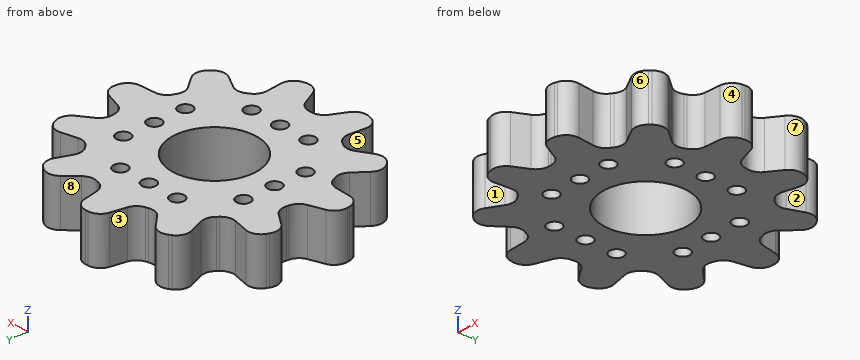
from build123d import *

# Parameters (mm, degrees)
ESBO_O1_R                = 4.5
ESBO_O1_R_2              = 0.75
RESSALTO_EXTRUS_O1_DEPTH = 5


with BuildPart() as part:
    # Esboço1 → Ressalto-extrusão1 (new body)
    with BuildSketch(Plane.XY):
        with BuildLine():
            Line((4.514334386, 10.407189323), (5.686971288, 11.63699072))
            ThreePointArc((5.686971288, 11.63699072), (6.526679908, 12.060076339), (7.444654683, 11.856522115))
            ThreePointArc((7.444654683, 11.856522115), (7.568971444, 11.77754946), (7.692450547, 11.697273382))
            ThreePointArc((7.692450547, 11.697273382), (8.258950485, 10.946813637), (8.222925837, 10.007231691))
            Line((8.222925837, 10.007231691), (7.591390112, 8.429685683))
            ThreePointArc((7.591390112, 8.429685683), (7.512037525, 7.668211946), (7.845097462, 6.978857056))
            ThreePointArc((7.845097462, 6.978857056), (7.935370531, 6.876037706), (8.024296131, 6.772050768))
            ThreePointArc((8.024296131, 6.772050768), (8.65923501, 6.344275472), (9.424251093, 6.314451352))
            Line((9.424251093, 6.314451352), (11.075616863, 6.715050749))
            ThreePointArc((11.075616863, 6.715050749), (12.010762061, 6.616992265), (12.672961861, 5.949456923))
            ThreePointArc((12.672961861, 5.949456923), (12.734847935, 5.815810182), (12.795324642, 5.681519805))
            ThreePointArc((12.795324642, 5.681519805), (12.866165546, 4.743919904), (12.327883333, 3.972969668))
            Line((12.327883333, 3.972969668), (10.94371591, 2.987287505))
            ThreePointArc((10.94371591, 2.987287505), (10.465276482, 2.389596282), (10.372770939, 1.629608249))
            ThreePointArc((10.372770939, 1.629608249), (10.39312514, 1.494305802), (10.411714532, 1.358749614))
            ThreePointArc((10.411714532, 1.358749614), (10.714586321, 0.655608259), (11.342034667, 0.216919693))
            Line((11.342034667, 0.216919693), (12.94783234, -0.338870389))
            ThreePointArc((12.94783234, -0.338870389), (13.681512123, -0.926940099), (13.877693191, -1.846518805))
            ThreePointArc((13.877693191, -1.846518805), (13.857500186, -1.992407736), (13.835773571, -2.138076166))
            ThreePointArc((13.835773571, -2.138076166), (13.388463955, -2.96513488), (12.518824975, -3.322682154))
            Line((12.518824975, -3.322682154), (10.82148923, -3.403553348))
            ThreePointArc((10.82148923, -3.403553348), (10.095864099, -3.647699318), (9.607162934, -4.237029663))
            ThreePointArc((9.607162934, -4.237029663), (9.551135951, -4.361857637), (9.493487134, -4.485944943))
            ThreePointArc((9.493487134, -4.485944943), (9.368132181, -5.241209943), (9.658802374, -5.949482436))
            Line((9.658802374, -5.949482436), (10.709202535, -7.285202572))
            ThreePointArc((10.709202535, -7.285202572), (11.008478755, -8.176575531), (10.676354988, -9.05623786))
            ThreePointArc((10.676354988, -9.05623786), (10.580494041, -9.168050275), (10.48346215, -9.278848062))
            ThreePointArc((10.48346215, -9.278848062), (9.660019656, -9.73278029), (8.735128141, -9.563405868))
            Line((8.735128141, -9.563405868), (7.263516181, -8.713790062))
            ThreePointArc((7.263516181, -8.713790062), (6.521086199, -8.526876158), (5.791348577, -8.758440595))
            ThreePointArc((5.791348577, -8.758440595), (5.676728583, -8.833162095), (5.56114465, -8.906383676))
            ThreePointArc((5.56114465, -8.906383676), (5.047362265, -9.473981021), (4.908968572, -10.226965929))
            Line((4.908968572, -10.226965929), (5.070476592, -11.918534414))
            ThreePointArc((5.070476592, -11.918534414), (4.840331165, -12.830206005), (4.085349512, -13.390665382))
            ThreePointArc((4.085349512, -13.390665382), (3.944255796, -13.432901631), (3.802725568, -13.473651259))
            ThreePointArc((3.802725568, -13.473651259), (2.864587371, -13.410336727), (2.178089842, -12.767815792))
            Line((2.178089842, -12.767815792), (1.399428066, -11.257459999))
            ThreePointArc((1.399428066, -11.257459999), (0.875909507, -10.698830065), (0.136821968, -10.499108522))
            ThreePointArc((0.136821968, -10.499108522), (0, -10.5), (-0.136821968, -10.499108522))
            ThreePointArc((-0.136821968, -10.499108522), (-0.875909507, -10.698830065), (-1.399428066, -11.257459999))
            Line((-1.399428066, -11.257459999), (-2.178089842, -12.767815792))
            ThreePointArc((-2.178089842, -12.767815792), (-2.864587371, -13.410336727), (-3.802725568, -13.473651259))
            ThreePointArc((-3.802725568, -13.473651259), (-3.944255796, -13.432901631), (-4.085349512, -13.390665382))
            ThreePointArc((-4.085349512, -13.390665382), (-4.840331165, -12.830206005), (-5.070476592, -11.918534414))
            Line((-5.070476592, -11.918534414), (-4.908968572, -10.226965929))
            ThreePointArc((-4.908968572, -10.226965929), (-5.047362265, -9.473981021), (-5.56114465, -8.906383676))
            ThreePointArc((-5.56114465, -8.906383676), (-5.676728583, -8.833162095), (-5.791348577, -8.758440595))
            ThreePointArc((-5.791348577, -8.758440595), (-6.521086199, -8.526876158), (-7.263516181, -8.713790062))
            Line((-7.263516181, -8.713790062), (-8.735128141, -9.563405868))
            ThreePointArc((-8.735128141, -9.563405868), (-9.660019656, -9.73278029), (-10.48346215, -9.278848062))
            ThreePointArc((-10.48346215, -9.278848062), (-10.580494041, -9.168050275), (-10.676354988, -9.05623786))
            ThreePointArc((-10.676354988, -9.05623786), (-11.008478755, -8.176575531), (-10.709202535, -7.285202572))
            Line((-10.709202535, -7.285202572), (-9.658802374, -5.949482436))
            ThreePointArc((-9.658802374, -5.949482436), (-9.368132181, -5.241209943), (-9.493487134, -4.485944943))
            ThreePointArc((-9.493487134, -4.485944943), (-9.551135951, -4.361857637), (-9.607162934, -4.237029663))
            ThreePointArc((-9.607162934, -4.237029663), (-10.095864099, -3.647699318), (-10.82148923, -3.403553348))
            Line((-10.82148923, -3.403553348), (-12.518824975, -3.322682154))
            ThreePointArc((-12.518824975, -3.322682154), (-13.388463955, -2.96513488), (-13.835773571, -2.138076166))
            ThreePointArc((-13.835773571, -2.138076166), (-13.857500186, -1.992407736), (-13.877693191, -1.846518805))
            ThreePointArc((-13.877693191, -1.846518805), (-13.681512123, -0.926940099), (-12.94783234, -0.338870389))
            Line((-12.94783234, -0.338870389), (-11.342034667, 0.216919693))
            ThreePointArc((-11.342034667, 0.216919693), (-10.714586321, 0.655608259), (-10.411714532, 1.358749614))
            ThreePointArc((-10.411714532, 1.358749614), (-10.39312514, 1.494305802), (-10.372770939, 1.629608249))
            ThreePointArc((-10.372770939, 1.629608249), (-10.465276482, 2.389596282), (-10.94371591, 2.987287505))
            Line((-10.94371591, 2.987287505), (-12.327883333, 3.972969668))
            ThreePointArc((-12.327883333, 3.972969668), (-12.866165546, 4.743919904), (-12.795324642, 5.681519805))
            ThreePointArc((-12.795324642, 5.681519805), (-12.734847935, 5.815810182), (-12.672961861, 5.949456923))
            ThreePointArc((-12.672961861, 5.949456923), (-12.010762061, 6.616992265), (-11.075616863, 6.715050749))
            Line((-11.075616863, 6.715050749), (-9.424251093, 6.314451352))
            ThreePointArc((-9.424251093, 6.314451352), (-8.65923501, 6.344275472), (-8.024296131, 6.772050768))
            ThreePointArc((-8.024296131, 6.772050768), (-7.935370531, 6.876037706), (-7.845097462, 6.978857056))
            ThreePointArc((-7.845097462, 6.978857056), (-7.512037525, 7.668211946), (-7.591390112, 8.429685683))
            Line((-7.591390112, 8.429685683), (-8.222925837, 10.007231691))
            ThreePointArc((-8.222925837, 10.007231691), (-8.258950485, 10.946813637), (-7.692450547, 11.697273382))
            ThreePointArc((-7.692450547, 11.697273382), (-7.568971444, 11.77754946), (-7.444654683, 11.856522115))
            ThreePointArc((-7.444654683, 11.856522115), (-6.526679908, 12.060076339), (-5.686971288, 11.63699072))
            Line((-5.686971288, 11.63699072), (-4.514334386, 10.407189323))
            ThreePointArc((-4.514334386, 10.407189323), (-3.854637767, 10.018680048), (-3.089220405, 10.035273653))
            ThreePointArc((-3.089220405, 10.035273653), (-2.958191847, 10.074676223), (-2.826660972, 10.112368059))
            ThreePointArc((-2.826660972, 10.112368059), (-2.173779732, 10.512224498), (-1.828851593, 11.195718217))
            Line((-1.828851593, 11.195718217), (-1.507247489, 12.864268361))
            ThreePointArc((-1.507247489, 12.864268361), (-1.029577, 13.674171387), (-0.147277756, 13.999225309))
            ThreePointArc((-0.147277756, 13.999225309), (0, 14), (0.147277756, 13.999225309))
            ThreePointArc((0.147277756, 13.999225309), (1.029577, 13.674171387), (1.507247489, 12.864268361))
            Line((1.507247489, 12.864268361), (1.828851593, 11.195718217))
            ThreePointArc((1.828851593, 11.195718217), (2.173779732, 10.512224498), (2.826660972, 10.112368059))
            ThreePointArc((2.826660972, 10.112368059), (2.958191847, 10.074676223), (3.089220405, 10.035273653))
            ThreePointArc((3.089220405, 10.035273653), (3.854637767, 10.018680048), (4.514334386, 10.407189323))
        make_face()
        Circle(ESBO_O1_R, mode=Mode.SUBTRACT)
        with Locations((3.4, 7.18)):
            Circle(ESBO_O1_R_2, mode=Mode.SUBTRACT)
        with Locations((0, 7.18)):
            Circle(ESBO_O1_R_2, mode=Mode.SUBTRACT)
        with Locations((-3.4, 7.18)):
            Circle(ESBO_O1_R_2, mode=Mode.SUBTRACT)
        with Locations((7.18, -3.4)):
            Circle(ESBO_O1_R_2, mode=Mode.SUBTRACT)
        with Locations((7.18, 0)):
            Circle(ESBO_O1_R_2, mode=Mode.SUBTRACT)
        with Locations((7.18, 3.4)):
            Circle(ESBO_O1_R_2, mode=Mode.SUBTRACT)
        with Locations((-3.4, -7.18)):
            Circle(ESBO_O1_R_2, mode=Mode.SUBTRACT)
        with Locations((0, -7.18)):
            Circle(ESBO_O1_R_2, mode=Mode.SUBTRACT)
        with Locations((3.4, -7.18)):
            Circle(ESBO_O1_R_2, mode=Mode.SUBTRACT)
        with Locations((-7.18, 3.4)):
            Circle(ESBO_O1_R_2, mode=Mode.SUBTRACT)
        with Locations((-7.18, 0)):
            Circle(ESBO_O1_R_2, mode=Mode.SUBTRACT)
        with Locations((-7.18, -3.4)):
            Circle(ESBO_O1_R_2, mode=Mode.SUBTRACT)
    extrude(amount=RESSALTO_EXTRUS_O1_DEPTH)


solid = part.part
Input: part model. Units: mm. Frame: model coordinates. Face numbers are marked on the shaded views. A direction names the side the tool comes from. Give positions to 0.01 mm unless a question says otherwise; leave off trailing zeros. Order: outer loops, then holes, each group sorted by start corner. A loop starts at its lowest first (then second) coordinate and runs counter-clockwise, first axis right, second up.
Q1. Contact query for flat-ended pins moving along their axis: pin 1 Ø3 at (y, z) = (-4, 2.5) entering from +X; pin 2 Ø1.5 at (x, z) = (5.5, 4.5) entering from +Y; pin 3 Ø1 at (x, z) = (-10.5, 1) entering from +Y. Output: stop coordinate, or through.
Checked values:
pin 1: stops at x = 13.73
pin 2: stops at y = 12
pin 3: stops at y = 6.7
Q2. Section B-B on z = 3.55. State how many separate pieces and enclosed holes the cut face has, and give its area (3 significant figures).
Checked values:
separate pieces: 1
enclosed holes: 13
area: 387 mm2
Q3. Section A-A on y = 2. Output: boundary loops of the cut face in (x, z).
Checked values:
outline: (-10.36, 0) - (-4.03, 0) - (-4.03, 5) - (-10.36, 5) - close; (4.03, 0) - (10.36, 0) - (10.36, 5) - (4.03, 5) - close
Q4. Set-up query: the marked faces 1, 2, 3, 4 and 5. Return all of +Z, -Z, +X, -X, +Y, -Y with unobstructed straight access to the full face (end or side cutting, diameter ignored); none if empty.
Checked values:
face 1: +Z, -Z, -Y
face 2: +Z, -Z, +X
face 3: +Z, -Z, +Y
face 4: +Z, -Z, +X, -Y
face 5: +Z, -Z, -X
Q5. Draft query along Y for the marked faces 6, 7 and 8. Return one class per face: +Y half, -Y half, draft (parallel to the pull), parting line (faces both ways), or undercut.
Checked values:
face 6: -Y half
face 7: undercut
face 8: +Y half
Q6. Ray query, probe 1 along Y at (x, z) = (0, 2.85); probe 2 along Y at (x, z) = (-3.4, 2); probe 3 along X at (y, z) = (-0.5, 3.4). Return the intervals inside material, ascending.
Checked values:
probe 1: y = -10.5 to -7.93, -6.43 to -4.5, 4.5 to 6.43, 7.93 to 14
probe 2: y = -13.53 to -7.93, -6.43 to -2.95, 2.95 to 6.43, 7.93 to 9.98
probe 3: x = -13.27 to -7.74, -6.62 to -4.47, 4.47 to 6.62, 7.74 to 13.27
